Check sheet for the modelled part. Datum: model origin and axes. Units: mm. Face numbers are marked on the shaded views. A direction names the side the tool comes from. Round coordinates to 2 decimals unless told otherwise and drop trailing zeros. Loops run counter-clockwise (first coordinate to the right, second up) from the corner with the lowest first, then second, coordinate; pieces in that order, holes last. Notation, with made-up numbers: (52.25, 5.25) - (86.25, 5.25) arc R14 ccw to (86.25, 30.25) - close; hole circle Ø6 at (24, 9.25). An arc over 180 degrees is marked (long way). Put each result on its own line as item: value. Start each with the question number.
```python
from build123d import *

# Parameters (mm, degrees)
BOSS_EXTRUDE1_DEPTH       = 19.05
SKETCH2_W                 = 25.4
SKETCH2_H                 = 31.75
SKETCH2_W_2               = 31.75
SKETCH2_H_2               = 25.4
CUT_EXTRUDE1_DEPTH        = 19.05
FILLET1_R                 = 25.4
FILLET2_R                 = 6.35
BODY_MOVE_COPY1_OUTLINE_W = 31.75
BODY_MOVE_COPY1_OUTLINE_H = 25.4
BODY_MOVE_COPY1_DEPTH     = 19.05
BODY_MOVE_COPY1_2_DEPTH   = 19.05


# Read off the part's stored shape, not the designer's step: Body-Move/Copy1
with BuildPart() as part:
    # Sketch1 → Boss-Extrude1 (new body)
    with BuildSketch(Plane(origin=(0, 0, 0), x_dir=(1, 0, 0), z_dir=(0, 1, 0))):
        Polygon((104.775, 223.510378542), (104.775, 293.360378542), (180.975, 293.360378542), (180.975, 223.510378542), (223.510378542, 223.510378542), (0, 0), (0, 42.535378542), (-69.85, 42.535378542), (-69.85, 118.735378542), (0, 118.735378542), (0, 188.585378542), (34.925, 188.585378542), (34.925, 223.510378542), align=None)
    extrude(amount=BOSS_EXTRUDE1_DEPTH)

    # Sketch2 → Cut-Extrude1 (cut)
    with BuildSketch(Plane(origin=(0, 19.05, 0), x_dir=(1, 0, 0), z_dir=(0, 1, 0))):
        with Locations((-30.48, 80.635378542)):
            Rectangle(SKETCH2_W, SKETCH2_H)
        with Locations((142.875, 253.990378542)):
            Rectangle(SKETCH2_W_2, SKETCH2_H_2)
    extrude(amount=-CUT_EXTRUDE1_DEPTH, mode=Mode.SUBTRACT)

    # Fillet1
    fillet1_edges = [part.edges().sort_by_distance(p)[0] for p in [
        (104.775, 9.525, -293.360378542),
        (180.975, 9.525, -293.360378542),
        (-69.85, 9.525, -42.535378542),
        (-69.85, 9.525, -118.735378542),
    ]]
    fillet(fillet1_edges, radius=FILLET1_R)

    # Fillet2
    fillet2_edges = [part.edges().sort_by_distance(p)[0] for p in [
        (223.510378542, 9.525, -223.510378542),
        (0, 9.525, 0),
        (0, 9.525, -188.585378542),
        (34.925, 9.525, -188.585378542),
        (34.925, 9.525, -223.510378542),
    ]]
    fillet(fillet2_edges, radius=FILLET2_R)

    # Body-Move/Copy1 outline → Body-Move/Copy1 (cut)
    # profile 1 of 2: a face of its own
    with BuildSketch(Plane(origin=(0, 0, 0), x_dir=(1, 0, 0), z_dir=(0, 1, 0))):
        with BuildLine():
            Line((122.509871939, 128.859871939), (125.684871939, 125.684871939))
            Line((125.684871939, 125.684871939), (212.670250482, 212.670250482))
            ThreePointArc((212.670250482, 212.670250482), (214.046757453, 219.590418338), (208.180122421, 223.510378542))
            Line((208.180122421, 223.510378542), (180.975, 223.510378542))
            Line((180.975, 223.510378542), (180.975, 267.960378542))
            ThreePointArc((180.975, 267.960378542), (173.535512243, 285.920890784), (155.575, 293.360378542))
            Line((155.575, 293.360378542), (130.175, 293.360378542))
            ThreePointArc((130.175, 293.360378542), (112.214487758, 285.920890784), (104.775, 267.960378542))
            Line((104.775, 267.960378542), (104.775, 223.510378542))
            Line((104.775, 223.510378542), (41.275, 223.510378542))
            ThreePointArc((41.275, 223.510378542), (36.784871939, 221.650506603), (34.925, 217.160378542))
            Line((34.925, 217.160378542), (34.925, 194.935378542))
            ThreePointArc((34.925, 194.935378542), (33.06512806, 190.445250481), (28.575, 188.585378542))
            Line((28.575, 188.585378542), (6.35, 188.585378542))
            ThreePointArc((6.35, 188.585378542), (1.859871939, 186.725506603), (0, 182.235378542))
            Line((0, 182.235378542), (0, 118.735378542))
            Line((0, 118.735378542), (-44.45, 118.735378542))
            ThreePointArc((-44.45, 118.735378542), (-62.410512242, 111.295890785), (-69.85, 93.335378542))
            Line((-69.85, 93.335378542), (-69.85, 67.935378542))
            ThreePointArc((-69.85, 67.935378542), (-62.410512242, 49.9748663), (-44.45, 42.535378542))
            Line((-44.45, 42.535378542), (0, 42.535378542))
            Line((0, 42.535378542), (0, 15.330256121))
            Line((0, 15.330256121), (14.746798487, 30.077054608))
            Line((14.746798487, 30.077054608), (-16.684097937, 61.507951031))
            ThreePointArc((-16.684097937, 61.507951031), (-18.126244186, 63.076488301), (-19.431850797, 64.760378542))
            Line((-19.431850797, 64.760378542), (-43.18, 64.760378542))
            Line((-43.18, 64.760378542), (-43.18, 96.510378542))
            Line((-43.18, 96.510378542), (-17.78, 96.510378542))
            Line((-17.78, 96.510378542), (-17.78, 96.261708161))
            ThreePointArc((-17.78, 96.261708161), (-17.241248642, 96.853979055), (-16.684097937, 97.428975516))
            Line((-16.684097937, 97.428975516), (1.276414305, 115.389487758))
            ThreePointArc((1.276414305, 115.389487758), (19.236926547, 122.828975516), (37.197438789, 115.389487758))
            Line((37.197438789, 115.389487758), (68.628335213, 83.958591334))
            Line((68.628335213, 83.958591334), (113.529615818, 128.859871939))
            ThreePointArc((113.529615818, 128.859871939), (118.019743879, 130.719743879), (122.509871939, 128.859871939))
        make_face()
        with Locations((142.875, 253.990378542)):
            Rectangle(BODY_MOVE_COPY1_OUTLINE_W, BODY_MOVE_COPY1_OUTLINE_H, mode=Mode.SUBTRACT)
    # profile 2 of 2: a face of its own
    with BuildSketch(Plane(origin=(0, 0, 0), x_dir=(1, 0, 0), z_dir=(0, 1, 0))):
        Polygon((40.340528432, 80.815501692), (22.38001619, 98.776013934), (-0.070624113, 76.325373631), (17.889888129, 58.364861389), align=None)
    extrude(amount=BODY_MOVE_COPY1_DEPTH, mode=Mode.SUBTRACT)

    # Body-Move_Copy1 2 outline → Body-Move_Copy1 2 (add)
    # profile 1 of 2: a face of its own
    with BuildSketch(Plane(origin=(0, 0, 0), x_dir=(1, 0, 0), z_dir=(0, 1, 0))):
        with BuildLine():
            Line((216.802561211, 83.958591334), (171.901280605, 128.859871939))
            ThreePointArc((171.901280605, 128.859871939), (167.411152544, 130.719743879), (162.921024484, 128.859871939))
            Line((162.921024484, 128.859871939), (147.205576272, 113.144423728))
            ThreePointArc((147.205576272, 113.144423728), (142.715448211, 111.284551788), (138.225320151, 113.144423728))
            Line((138.225320151, 113.144423728), (125.684871939, 125.684871939))
            Line((125.684871939, 125.684871939), (10.840128061, 10.840128061))
            ThreePointArc((10.840128061, 10.840128061), (3.919960205, 9.46362109), (0, 15.330256121))
            Line((0, 15.330256121), (-4.490128061, 10.840128061))
            ThreePointArc((-4.490128061, 10.840128061), (-5.866635031, 3.919960205), (0, 0))
            Line((0, 0), (285.430896424, 0))
            ThreePointArc((285.430896424, 0), (291.297531455, 3.919960205), (289.921024484, 10.840128061))
            Line((289.921024484, 10.840128061), (270.684097937, 30.077054608))
            Line((270.684097937, 30.077054608), (302.114994361, 61.507951031))
            ThreePointArc((302.114994361, 61.507951031), (309.554482119, 79.468463273), (302.114994361, 97.428975516))
            Line((302.114994361, 97.428975516), (284.154482119, 115.389487758))
            ThreePointArc((284.154482119, 115.389487758), (266.193969876, 122.828975516), (248.233457634, 115.389487758))
            Line((248.233457634, 115.389487758), (216.802561211, 83.958591334))
        make_face()
        Polygon((245.090367992, 80.815501692), (263.050880234, 98.776013934), (285.501520537, 76.325373631), (267.541008295, 58.364861389), align=None, mode=Mode.SUBTRACT)
    # profile 2 of 2: a face of its own
    with BuildSketch(Plane(origin=(0, 0, 0), x_dir=(1, 0, 0), z_dir=(0, 1, 0))):
        with BuildLine():
            ThreePointArc((-17.78, 96.261708161), (-24.088736474, 80.798548227), (-19.431850797, 64.760378542))
            Line((-19.431850797, 64.760378542), (-17.78, 64.760378542))
            Line((-17.78, 64.760378542), (-17.78, 96.261708161))
        make_face()
    extrude(amount=BODY_MOVE_COPY1_2_DEPTH)


solid = part.part
```
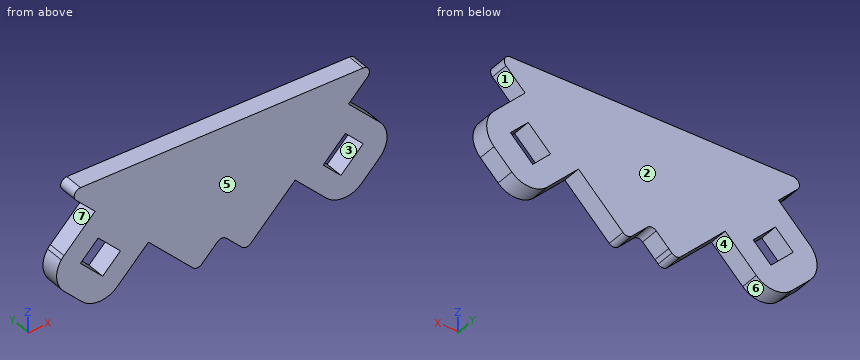
Q1. Cross-section at C-C on x = 65.5. Enter the section's corners in (y, z).
Q2. Cross-section at A-A on y = 3.5. State how many separate pieces and enclosed holes the cut face has, and give its area (3 significant figures).
Q3. Material ranges on line 1 (Z direction, x = 271, y = 13.25); line 2 (X direction, y = 5.25, z = -112.5); line 3 (X direction, y = 13, z = -100.5), recorded low to high. Write a range as from..to.
Q4. Set-up check for the marked faces 1, 2, 3 and 4: record each of +Z, -Z, +X, -X, +Y, -Y from which the full face is reachable in a straight line by a thin tool's end or side.
Q5. Cross-section at B-B on z = -104. Enter the section's corners in (x, y).
Q6. Depth check by flat-ended pin: pin 1 Ø8 at (x, y) = (9.5, 15.5) entering from -Z; pin 2 Ø10 at (x, y) = (202.5, 14.5) entering from -Z; pin 3 Ø6 at (y, z) = (11.5, -31.5) entering from -X. Enter the tip coordinate at first touch or a pass-through.
Q7. Cross-section at D-D on x = 239.5. Enter the section's corners in (y, z).
Q8. Draft check along X on the marked faces 5, 6 and 7. Enter one of: +X half, -X half, draft (parallel to the pull), parting line (faces both ways), or undercut.
Answer list:
1. outline: (0, -87.09) - (19.05, -87.09) - (19.05, 0) - (0, 0) - close
2. separate pieces: 1
2. enclosed holes: 2
2. area: 32,100 mm2
3. line 1: z = -122.37..-90.83, -61.82..-30.39, -29.76..0
3. line 2: x = -1.61..40.09, 97.17..138.98, 146.45..188.26, 245.34..287.04
3. line 3: x = -13.61..52.09, 85.17..200.26, 233.34..299.04
4. face 1: +X, +Y, -Y
4. face 2: +Z, -Z, +X, -X, +Y
4. face 3: +Y, -Y
4. face 4: -Z, +Y, -Y
5. outline: (-10.11, 0) - (48.59, 0) - (48.59, 19.05) - (-10.11, 19.05) - close; (88.67, 0) - (196.76, 0) - (196.76, 19.05) - (88.67, 19.05) - close; (236.84, 0) - (295.54, 0) - (295.54, 19.05) - (236.84, 19.05) - close
6. pin 1: stops at z = -122.17
6. pin 2: stops at z = -103.26
6. pin 3: stops at x = 10.32
7. outline: (0, -106.66) - (19.05, -106.66) - (19.05, 0) - (0, 0) - close
8. face 5: draft
8. face 6: undercut
8. face 7: -X half
